Verification items for the finished model (mm, model axes). Face numbers are marked on the shaded views. Give positions to 0.01 mm unless a question says otherwise; leave off trailing zeros. Order: outer loops, then holes, each group sorted by start corner. A loop starts at its lowest first (then second) coordinate and runs counter-clockwise, first axis right, second up. Notation, with made-up numbers: (44, -12) - (82, -12) arc R19 ccw to (82, -7) - close; hole circle Ø5 at (-25, 70). An arc over 180 degrees is marked (long way). Answer as a JSON object with one key per item and string values. Group by question number.
(1) Thickness scan on line 1 (X direction, y = 2, z = -60); line 2 (X direction, y = 2.1, z = -18); line 3 (X direction, y = 1.75, z = 132). Record the ranges inside material, lowest first.
(2) Mould release check, pull along Y, two halves, no side actions. Record for the marked faces 1 and 2: +Y half, -Y half, draft (parallel to the pull), parting line (faces both ways), or undercut.
(3) Section check A-A (z = -107). Record the boundary of the cut face in (x, y), then the cut area to 3 significant figures.
(4) Depth check by flat-ended pin: pin 1 Ø2.5 at (x, z) = (67.66, -82.18) entering from -Y; pin 2 Ø1.5 at (y, z) = (1.5, 98.5) entering from +X; pin 3 Ø0.9 at (y, z) = (1, 102) entering from -X; pin 4 Ø0.9 at (x, y) = (-151, 1) entering from +Z. Enter the tip coordinate at first touch or a pass-through.
(5) Section check B-B (y = 2.05). Count the separate pieces of the cut face and the enclosed holes in it, then the cut area to 3 significant figures.
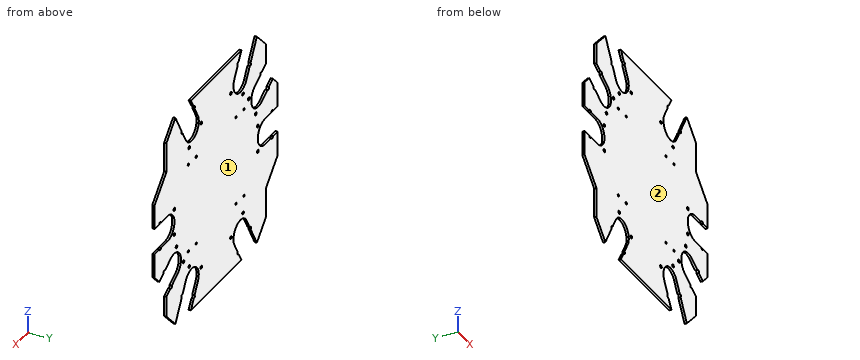
```python
from build123d import *

# Parameters (mm, degrees)
BOSS_EXTRUDE1_DEPTH  = 3
SKETCH2_R            = 2.05
HEXCUT1_DEPTH        = 3
SKETCH5_R            = 1.55
CUT_EXTRUDE2_DEPTH   = 3
LPATTERN1_COUNT      = 2
LPATTERN1_PITCH      = 120
LPATTERN1_COUNT_DIR2 = 2
LPATTERN1_PITCH_DIR2 = 120
SKETCH6_R            = 2.05
QUADCUT1_DEPTH       = 3
CUT_EXTRUDE3_DEPTH   = 3
CUT_EXTRUDE4_DEPTH   = 3


with BuildPart() as part:
    # Sketch1 → Boss-Extrude1 (new body)
    with BuildSketch(Plane(origin=(0, 0, 0), x_dir=(1, 0, 0), z_dir=(0, 1, 0))):
        Polygon((-100, 145), (-125, 120), (-125, 80), (-155, 50), (-155, -50), (-125, -80), (-125, -120), (-100, -145), (100, -145), (125, -120), (125, -80), (155, -50), (155, 50), (125, 80), (125, 120), (100, 145), align=None)
    extrude(amount=BOSS_EXTRUDE1_DEPTH)

    # Sketch2 → HexCut1 (cut)
    with BuildSketch(Plane(origin=(0, 3, 0), x_dir=(1, 0, 0), z_dir=(0, 1, 0))):
        with Locations(Location((55.344555434, 130.859581934, 0), (0, 0, 270))):
            Circle(SKETCH2_R)
        with Locations(Location((37.344555434, 99.682667397, 0), (0, 0, 270))):
            Circle(SKETCH2_R)
        with Locations(Location((37.344555434, -99.682667397, 0), (0, 0, 270))):
            Circle(SKETCH2_R)
        with Locations(Location((55.344555434, -130.859581934, 0), (0, 0, 270))):
            Circle(SKETCH2_R)
        with Locations(Location((105, 17.5, 0), (0, 0, 270))):
            Circle(SKETCH2_R)
        with Locations(Location((141, 17.5, 0), (0, 0, 270))):
            Circle(SKETCH2_R)
        with Locations(Location((105, -17.5, 0), (0, 0, 270))):
            Circle(SKETCH2_R)
        with Locations(Location((141, -17.5, 0), (0, 0, 270))):
            Circle(SKETCH2_R)
        with Locations(Location((85.655444566, -113.359581934, 0), (0, 0, 270))):
            Circle(SKETCH2_R)
        with Locations(Location((67.655444566, -82.182667397, 0), (0, 0, 270))):
            Circle(SKETCH2_R)
        with Locations(Location((85.655444566, 113.359581934, 0), (0, 0, 270))):
            Circle(SKETCH2_R)
        with Locations(Location((67.655444566, 82.182667397, 0), (0, 0, 270))):
            Circle(SKETCH2_R)
    hexcut1 = extrude(amount=-HEXCUT1_DEPTH, mode=Mode.SUBTRACT)

    # HexCut2: HexCut1 across plane
    add(hexcut1.mirror(Plane(origin=(0, 0, 0), x_dir=(0, 0, 1), z_dir=(1, 0, 0))), mode=Mode.SUBTRACT)

    # Sketch5 → Cut-Extrude2 (cut)
    with BuildSketch(Plane(origin=(0, 3, 0), x_dir=(1, 0, 0), z_dir=(0, 1, 0))):
        with Locations(Location((50, 60, 0), (0, 0, 270))):
            Circle(SKETCH5_R)
        with Locations(Location((70, 60, 0), (0, 0, 270))):
            Circle(SKETCH5_R)
    cut_extrude2 = extrude(amount=-CUT_EXTRUDE2_DEPTH, mode=Mode.SUBTRACT)

    # LPattern1: Cut-Extrude2 2 × 2
    with Locations(*[(-j * LPATTERN1_PITCH_DIR2, 0, i * LPATTERN1_PITCH) for i in range(LPATTERN1_COUNT) for j in range(LPATTERN1_COUNT_DIR2) if (i, j) != (0, 0)]):
        add(cut_extrude2, mode=Mode.SUBTRACT)

    # Sketch6 → QuadCut1 (cut)
    with BuildSketch(Plane(origin=(0, 3, 0), x_dir=(1, 0, 0), z_dir=(0, 1, 0))):
        with Locations(Location((99.682667397, 37.344555434, 0), (0, 0, 270))):
            Circle(SKETCH6_R)
        with Locations(Location((130.859581934, 55.344555434, 0), (0, 0, 270))):
            Circle(SKETCH6_R)
        with Locations(Location((113.359581934, 85.655444566, 0), (0, 0, 270))):
            Circle(SKETCH6_R)
        with Locations(Location((82.182667397, 67.655444566, 0), (0, 0, 270))):
            Circle(SKETCH6_R)
    quadcut1 = extrude(amount=-QUADCUT1_DEPTH, mode=Mode.SUBTRACT)

    # Mirror1: QuadCut1 across plane
    add(quadcut1.mirror(Plane(origin=(0, 0, 0), x_dir=(0.5000000000000011, 0, 0.8660254037844378), z_dir=(0.8660254037844379, 0, -0.5000000000000012))), mode=Mode.SUBTRACT)

    # Sketch7 → Cut-Extrude3 (cut)
    with BuildSketch(Plane(origin=(0, 3, 0), x_dir=(1, 0, 0), z_dir=(0, 1, 0))):
        with BuildLine():
            Line((45.994555434, 114.664906883), (83.494555434, 179.616812167))
            Line((83.494555434, 179.616812167), (113.805444566, 162.116812167))
            Line((113.805444566, 162.116812167), (76.305444566, 97.164906883))
            ThreePointArc((76.305444566, 97.164906883), (52.4, 90.759462317), (45.994555434, 114.664906883))
        make_face()
        with BuildLine():
            Line((45.994555434, -114.664906883), (83.494555434, -179.616812167))
            Line((83.494555434, -179.616812167), (113.805444566, -162.116812167))
            Line((113.805444566, -162.116812167), (76.305444566, -97.164906883))
            ThreePointArc((76.305444566, -97.164906883), (52.4, -90.759462317), (45.994555434, -114.664906883))
        make_face()
        with BuildLine():
            Line((122.3, 17.5), (162.3, 17.5))
            Line((162.3, 17.5), (162.3, -17.5))
            Line((162.3, -17.5), (122.3, -17.5))
            ThreePointArc((122.3, -17.5), (104.8, 0), (122.3, 17.5))
        make_face()
    cut_extrude3 = extrude(amount=-CUT_EXTRUDE3_DEPTH, mode=Mode.SUBTRACT)

    # Mirror2: Cut-Extrude3 across plane
    add(cut_extrude3.mirror(Plane(origin=(0, 0, 0), x_dir=(0, 0, 1), z_dir=(1, 0, 0))), mode=Mode.SUBTRACT)

    # Sketch8 → Cut-Extrude4 (cut)
    with BuildSketch(Plane(origin=(0, 3, 0), x_dir=(1, 0, 0), z_dir=(0, 1, 0))):
        with BuildLine():
            Line((97.164906883, 76.305444566), (131.805923034, 96.305444566))
            Line((131.805923034, 96.305444566), (149.305923034, 65.994555434))
            Line((149.305923034, 65.994555434), (114.664906883, 45.994555434))
            ThreePointArc((114.664906883, 45.994555434), (90.759462317, 52.4), (97.164906883, 76.305444566))
        make_face()
    cut_extrude4 = extrude(amount=-CUT_EXTRUDE4_DEPTH, mode=Mode.SUBTRACT)

    # Mirror3: Cut-Extrude4 across plane
    add(cut_extrude4.mirror(Plane(origin=(0, 0, 0), x_dir=(0.5000000000000011, 0, 0.8660254037844378), z_dir=(0.8660254037844379, 0, -0.5000000000000012))), mode=Mode.SUBTRACT)


solid = part.part
```
Solutions:
{
 "1": {"line 1": "x = -145 to -71.55, -68.45 to -51.55, -48.45 to 48.45, 51.55 to 68.45, 71.55 to 88.45, 138.92 to 145", "line 2": "x = -155 to -142.99, -139.01 to -106.99, -103.01 to 103.01, 106.99 to 139.01, 142.99 to 155", "line 3": "x = -113 to -96.42, -53.64 to 53.64, 96.42 to 113"},
 "2": {"face 1": "+Y half", "face 2": "-Y half"},
 "3": {"outline": "(-125, 0) - (-81.98, 0) - (-81.98, 3) - (-125, 3) - close; (-43.68, 0) - (43.68, 0) - (43.68, 3) - (-43.68, 3) - close; (81.98, 0) - (125, 0) - (125, 3) - (81.98, 3) - close", "area": "520 mm2"},
 "4": {"pin 1": "passes through", "pin 2": "stops at x = 125", "pin 3": "stops at x = -125", "pin 4": "stops at z = 54.45"},
 "5": {"separate pieces": "1", "enclosed holes": "24", "area": "64,200 mm2"}
}
